Work out the finished part from the listing and answer in its coordinate system (mm). A direction names the side the tool comes from. Coordinates: 2 decimals unless noted, no trailing zeros. Write each loop counter-clockwise with the first axis right and the second up, starting at its lowest first coordinate (ties: lowest second). Pieces come first, ordered by that corner, then holes. Notation, with made-up numbers: (-3.5, -7) - (11.5, -7) arc R13 ccw to (11.5, 16) - close; hole circle Ø3 at (28, 39.25). An arc over 180 degrees is marked (long way). Use one line per item in the form item = value. Start each with the question number.
Item 1: For faces 1 (the flat face through (0, -22.6, 3)), 2 (the flat face through (4.58, 0, 3)), 3 (the cylindrical face through (-20.227, 18.103, -0.837)), 4 (the flat face through (0, 22.6, 3)), 5 (the flat face through (0, 4.371, 9)), determine the directions among +Z, -Z, +X, -X, +Y, -Y from which every point of the face is accessible in a straight line to the end or side of a thin tool.
Item 2: Consider probe 1 along Y at (x, z) = (19.5, -1.05) (3 decimals); probe 2 along X at (y, z) = (-6, 2.75); probe 3 along Z at (x, y) = (-4, 16). Determine where each line is inside the solid, lowest interval first.
Item 3: A cutting plane is placed at B-B (y = 19.5). Write down the section's boundary in (x, z) (3 decimals).
Item 4: Given pin 1 (7 mm diameter, centred on y = -9, z = 4, fed in from -X); pin 2 (3 mm diameter, centred on x = 19.5, y = 19.5, fed in from +Z); pin 3 (0.9 mm diameter, centred on x = 0, z = 4, fed in from -Y); pin 4 (4 mm diameter, centred on x = 19.5, y = -19.5, fed in from +Z), each flat-ended and moving along its own axis, determine where each tip first touches the part or whether it passes through.
Item 5: A cutting plane is placed at D-D (y = 1). Write down the section's boundary in (x, z), then the cut area to 3 significant figures.
Item 6: A cutting plane is placed at A-A (z = 1.25). Write down the section's boundary in (x, y).
Item 7: A cutting plane is placed at C-C (x = -19.5). Write down the section's boundary in (y, z) (3 decimals), then the cut area to 3 significant figures.
from build123d import *

# Parameters (mm, degrees)
F0_W     = 51
F0_H     = 51
F3_DEPTH = 1.65
F4_D     = 3.15
F1_W     = 9.16
F1_H     = 45.2
F1_W_2   = 3.16
F1_H_2   = 37.2
F5_DEPTH = 6.45
F6_R     = 0.5
F2_W     = 1.8
F2_H     = 5
F7_DEPTH = 20
F8_SIZE  = 1


with BuildPart() as f3:
    # F0 (on Top) → F3 (new body)
    with BuildSketch(Plane.XY):
        Rectangle(F0_W, F0_H)
    extrude(amount=-F3_DEPTH)

    # F4 (through all)
    with Locations(Plane.XY):
        with Locations((-19.5, 19.5), (19.5, 19.5), (19.5, -19.5), (-19.5, -19.5)):
            Hole(F4_D / 2)

    # F1 (on Top) → F5 (join)
    with BuildSketch(Plane.XY):
        Rectangle(F1_W, F1_H)
        Rectangle(F1_W_2, F1_H_2, mode=Mode.SUBTRACT)
    extrude(amount=F5_DEPTH)

    # F6
    f6_edges = [f3.edges().sort_by_distance(p)[0] for p in [
        (4.58, 22.6, 3.225),
        (-4.58, 22.6, 3.225),
        (4.58, -22.6, 3.225),
        (-4.58, -22.6, 3.225),
        (4.58, 0, 6.45),
        (-4.58, 0, 6.45),
        (0, -22.6, 6.45),
        (0, 22.6, 6.45),
    ]]
    fillet(f6_edges, radius=F6_R)

    # F2 (on Top) → F7 (join)
    with BuildSketch(Plane.XY):
        with Locations((0, 6.87148829)):
            Rectangle(F2_W, F2_H)
    extrude(amount=F7_DEPTH)

    # F8
    f8_edges = [f3.edges().sort_by_distance(p)[0] for p in [
        (0, 4.371488, 20),
        (0, 9.371488, 20),
    ]]
    chamfer(f8_edges, length=F8_SIZE)


solid = f3.part
Answer:
q1.face_1 = +Z, +X, -X, -Y
q1.face_2 = +Z, +X, +Y, -Y
q1.face_3 = +Z, -Z
q1.face_4 = +Z, +X, -X, +Y
q1.face_5 = +Z
q2.probe_1 = -25.5 to -21.075, -17.925 to 17.925, 21.075 to 25.5
q2.probe_2 = -4.58 to -1.58, 1.58 to 4.58
q2.probe_3 = -1.65 to 6.45
q3.outline = (-25.5, -1.65) - (-21.075, -1.65) - (-21.075, 0) - (-25.5, 0) - close; (-17.925, -1.65) - (17.925, -1.65) - (17.925, 0) - (4.58, 0) - (4.58, 5.95) arc R0.5 ccw to (4.08, 6.45) - (-4.08, 6.45) arc R0.5 ccw to (-4.58, 5.95) - (-4.58, 0) - (-17.925, 0) - close; (21.075, -1.65) - (25.5, -1.65) - (25.5, 0) - (21.075, 0) - close
q4.pin_1 = -4.58
q4.pin_2 = through
q4.pin_3 = -22.6
q4.pin_4 = 0
q5.outline = (-25.5, -1.65) - (25.5, -1.65) - (25.5, 0) - (4.58, 0) - (4.58, 5.95) arc R0.5 ccw to (4.08, 6.45) - (1.58, 6.45) - (1.58, 0) - (-1.58, 0) - (-1.58, 6.45) - (-4.08, 6.45) arc R0.5 ccw to (-4.58, 5.95) - (-4.58, 0) - (-25.5, 0) - close
q5.area = 123 mm²
q6.outline = (-4.58, -22.1) arc R0.5 ccw to (-4.08, -22.6) - (4.08, -22.6) arc R0.5 ccw to (4.58, -22.1) - (4.58, 22.1) arc R0.5 ccw to (4.08, 22.6) - (-4.08, 22.6) arc R0.5 ccw to (-4.58, 22.1) - close; (-0.9, 4.37) - (0.9, 4.37) - (0.9, 9.37) - (-0.9, 9.37) - close; hole (-1.58, -18.6) - (1.58, -18.6) - (1.58, 18.6) - (-1.58, 18.6) - close
q7.outline = (-25.5, -1.65) - (-21.075, -1.65) - (-21.075, 0) - (-25.5, 0) - close; (-17.925, -1.65) - (17.925, -1.65) - (17.925, 0) - (-17.925, 0) - close; (21.075, -1.65) - (25.5, -1.65) - (25.5, 0) - (21.075, 0) - close
q7.area = 73.8 mm²
